Source: CAD feature listing. Evaluate the final solid. Frame: model axes, mm. A direction names the side the tool comes from. Give positions to 0.01 mm unless a question says otherwise; leave off trailing zeros. Order: outer loops, then holes, each group sorted by start corner. A loop starts at its lowest first (then second) coordinate and runs counter-clockwise, first axis right, second up.
1) Access query for faces 1 (the face through (1.97, 0.77, 16.37)), 2 (the face through (6, 1, 24.371)), 3 (the face through (27, 1, 14.814)). Directions: +Z, -Z, +X, -X, +Y, -Y. A direction counts if a zero-diameter tool reaches every point of the face in a straight line with its end or side. Return the directions, or none.
2) Section C-C, the plane x = 25.5. Return loops of the section in (y, z).
3) Section A-A, the plane y = 1. Return loops of the section in (x, z).
4) Draft query along X for faces 4 (the face through (0.724, 0.626, 0.764)), 5 (the face through (43.845, 1, 7)), 6 (the face through (3.48, 0.77, 17.93)). Return one class per face: released by +X, released by -X, zero draft, split by the parting line, or undercut.
5) Section B-B, the plane x = 6. Return loops of the section in (y, z).
6) Material intervals for line 1 (Z direction, x = 5, y = 1.2); line 2 (Z direction, x = 13, y = 0.75); line 3 (X direction, y = 0.3, z = 18.5), sorted ascending.
```python
from build123d import *

# Parameters (mm, degrees)
BOSS_EXTRUDE1_DEPTH = 1.27
CUT_EXTRUDE1_DEPTH  = 1.016


with BuildPart() as part:
    # Sketch1 → Boss-Extrude1 (new body)
    with BuildSketch(Plane(origin=(0, 0, 0), x_dir=(1, 0, 0), z_dir=(0, 1, 0))):
        with BuildLine():
            Line((2.54, 0), (41.304776771, 0))
            ThreePointArc((41.304776771, 0), (43.100827995, -0.743948776), (43.844776771, -2.54))
            Line((43.844776771, -2.54), (43.844776771, -12.274039018))
            ThreePointArc((43.844776771, -12.274039018), (43.100827995, -14.070090242), (41.304776771, -14.814039018))
            Line((41.304776771, -14.814039018), (11.827337603, -14.814039018))
            Line((11.827337603, -14.814039018), (11.827337603, -21.831483546))
            ThreePointArc((11.827337603, -21.831483546), (11.083388827, -23.62753477), (9.287337603, -24.371483546))
            Line((9.287337603, -24.371483546), (2.54, -24.371483546))
            ThreePointArc((2.54, -24.371483546), (0.743948776, -23.62753477), (0, -21.831483546))
            Line((0, -21.831483546), (0, -14.814039018))
            Line((0, -14.814039018), (0, -2.54))
            ThreePointArc((0, -2.54), (0.743948776, -0.743948776), (2.54, 0))
        make_face()
    extrude(amount=BOSS_EXTRUDE1_DEPTH)

    # Sketch2 → Cut-Extrude1 (cut)
    with BuildSketch(Plane(origin=(0, 1.27, 0), x_dir=(1, 0, 0), z_dir=(0, 1, 0))):
        with BuildLine():
            Line((8.125200896, -15.6495751), (3.744615047, -15.6495751))
            ThreePointArc((3.744615047, -15.6495751), (1.948563823, -16.393523876), (1.204615047, -18.1895751))
            Line((1.204615047, -18.1895751), (1.204615047, -20.061482924))
            ThreePointArc((1.204615047, -20.061482924), (1.948563823, -21.857534148), (3.744615047, -22.601482924))
            Line((3.744615047, -22.601482924), (8.125200896, -22.601482924))
            ThreePointArc((8.125200896, -22.601482924), (9.921252121, -21.857534148), (10.665200896, -20.061482924))
            Line((10.665200896, -20.061482924), (10.665200896, -18.1895751))
            ThreePointArc((10.665200896, -18.1895751), (9.921252121, -16.393523876), (8.125200896, -15.6495751))
        make_face()
        with BuildLine():
            Line((4.384925651, -17.552804899), (7.030054434, -17.552804899))
            ThreePointArc((7.030054434, -17.552804899), (7.928080046, -17.924779287), (8.300054434, -18.822804899))
            Line((8.300054434, -18.822804899), (8.300054434, -19.330205148))
            ThreePointArc((8.300054434, -19.330205148), (7.928080046, -20.228230761), (7.030054434, -20.600205148))
            Line((7.030054434, -20.600205148), (4.384925651, -20.600205148))
            ThreePointArc((4.384925651, -20.600205148), (3.486900039, -20.228230761), (3.114925651, -19.330205148))
            Line((3.114925651, -19.330205148), (3.114925651, -18.822804899))
            ThreePointArc((3.114925651, -18.822804899), (3.486900039, -17.924779287), (4.384925651, -17.552804899))
        make_face(mode=Mode.SUBTRACT)
    extrude(amount=-CUT_EXTRUDE1_DEPTH, mode=Mode.SUBTRACT)


solid = part.part
```
From the geometry:
1. face 1: +Y
1. face 2: +Z, +X, -X, +Y, -Y
1. face 3: +Z, +X, +Y, -Y
2. outline: (0, 0) - (1.27, 0) - (1.27, 14.81) - (0, 14.81) - close
3. outline: (0, 2.54) arc R2.54 ccw to (2.54, 0) - (41.3, 0) arc R2.54 ccw to (43.84, 2.54) - (43.84, 12.27) arc R2.54 ccw to (41.3, 14.81) - (11.83, 14.81) - (11.83, 21.83) arc R2.54 ccw to (9.29, 24.37) - (2.54, 24.37) arc R2.54 ccw to (0, 21.83) - close; (3.11, 18.82) arc R1.27 ccw to (4.38, 17.55) - (7.03, 17.55) arc R1.27 ccw to (8.3, 18.82) - (8.3, 19.33) arc R1.27 ccw to (7.03, 20.6) - (4.38, 20.6) arc R1.27 ccw to (3.11, 19.33) - close; hole (1.2, 18.19) arc R2.54 ccw to (3.74, 15.65) - (8.13, 15.65) arc R2.54 ccw to (10.67, 18.19) - (10.67, 20.06) arc R2.54 ccw to (8.13, 22.6) - (3.74, 22.6) arc R2.54 ccw to (1.2, 20.06) - close
4. face 4: released by -X
4. face 5: released by +X
4. face 6: undercut
5. outline: (0, 0) - (1.27, 0) - (1.27, 15.65) - (0.25, 15.65) - (0.25, 17.55) - (1.27, 17.55) - (1.27, 20.6) - (0.25, 20.6) - (0.25, 22.6) - (1.27, 22.6) - (1.27, 24.37) - (0, 24.37) - close
6. line 1: z = 0 to 15.65, 17.55 to 20.6, 22.6 to 24.37
6. line 2: z = 0 to 14.81
6. line 3: x = 0 to 1.2, 3.16 to 8.26, 10.67 to 11.83
